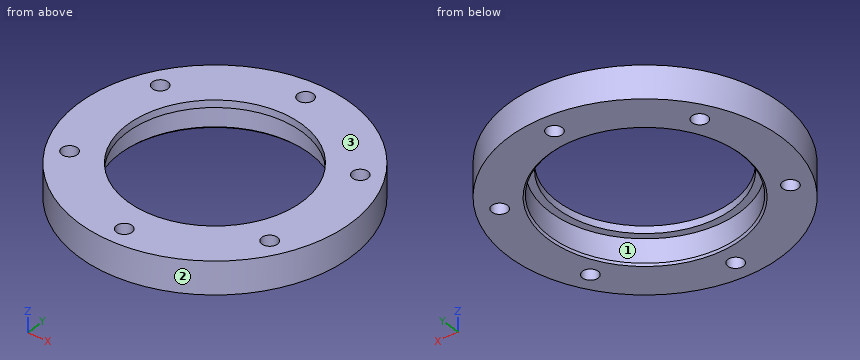
Autodesk Inventor part; units mm, degrees
ref_plane "YZ Plane" through (0, 0, 0) normal (1, 0, 0) x (0, 1, 0)
ref_plane "XZ Plane" through (0, 0, 0) normal (0, 1, 0) x (-1, 0, 0)
ref_plane "XY Plane" through (0, 0, 0) normal (0, 0, 1) x (1, 0, 0)
sketch "スケッチ1" plane through (0, 0, 0) normal (1, 0, 0) x (0, 1, 0)
  line L0 (24.1, 0) -> (24.1, -2)
  line L1 (24.1, -2) -> (26.1, -2)
  line L2 (26.1, -2) -> (26.1, -9)
  line L3 (26.1, -9) -> (37.5, -9)
  line L4 (37.5, -9) -> (37.5, 0)
  line L5 (37.5, 0) -> (24.1, 0)
  line L6 (0, -10.8) -> (0, 1.8)
  point P0 (0, 0)
  dimension "d0" = 26.1
  dimension "d1" = 37.5
  dimension "d2" = 7
  dimension "d3" = 2
  dimension "d4" = 2
revolve "回転1" add sketch "スケッチ1" angle 360 about axis through (0, 0, -10) along (0, 0, 1)
sketch "スケッチ2" plane through (0, 0, -9) normal (0, 0, -1) x (-1, 0, 0)
  circle A0 centre (0, 0) radius 32
  point P0 (0, 32)
  point P1 (-27.7128, 16)
  point P2 (-27.7128, -16)
  point P3 (0, -32)
  point P4 (27.7128, -16)
  point P5 (27.7128, 16)
  dimension "d6" = 64
  dimension "d9" = 360
hole "穴1" at (0, 32, -9) at (27.7128, 16, -9) at (27.7128, -16, -9) at (0, -32, -9) at (-27.7128, -16, -9) at (-27.7128, 16, -9) direction (0, 0, 1) diameter 4.3 end through all
chamfer "面取り1" distance 0.5 angle 45 1 edges at (0, -26.1, -9)
sketch "スケッチ3" plane through (0, 0, -9) normal (0, 0, -1) x (-1, 0, 0)
  circle A0 centre (-37.5, 0) radius 4.8
  circle A1 centre (0, 0) radius 37.5
  point P0 (-37.1928, 4.7902)
  point P1 (-37.1928, -4.7902)
  dimension "d18" = 9.6
properties part number "unit-base1" material "ABS プラスチック"
Geometry: final body of the model. Coordinates: model frame, mm. Face numbers are marked on the shaded views. Round coordinates to 2 decimals unless told otherwise and drop trailing zeros. Order: outer loops, then holes, each group sorted by start corner. A loop starts at its lowest first (then second) coordinate and runs counter-clockwise, first axis right, second up. Notation, with made-up numbers: M -22.75,17 L 23.25,17 A14 cw 23.25,33 Z; hole C -39.5,25 d8. An arc over 180 degrees is marked long. Use one line per item in the form item = value. Start each with the question number.
Q1. Cut plane D-D (y = -16). Count the separate pieces of the cut face and the enclosed holes in it, and give its area (3 significant figures).
Q2. Cut plane B-B (z = -6.5). Return loops of the section in (x, y).
Q3. Mould query, pull axis X, two halves, no side actions, for the marked faces 1, 2 and 3. Classes: +X half, -X half, draft (parallel to the pull), parting line (faces both ways), or undercut.
Q4. Cut plane C-C (y = -32). Return loops of the section in (x, z).
Q5. Material intervals for line 1 (Y direction, x = 0, z = -5); line 2 (X direction, y = -16, z = -2.25); line 3 (X direction, y = 0, z = -4.5), sorted ascending. Write a range as [from, to].
Q6. Cut plane A-A (y = 0). Return loops of the section in (x, z), and give its area (3 significant figures).
Q7. Pin query (flat end, axial travel): pin 1 Ø4 at (x, y) = (-27.71, 16) entering from +Z; pin 2 Ø4 at (x, z) = (-6.5, -1.5) entering from -Y; pin 3 Ø7 at (x, y) = (-27.71, -16) entering from -Z; pin 4 Ø1 at (x, z) = (9.5, -7) entering from -Y. Return the tip coordinate at first contact, or that it passes through.
Geometry results:
q1.separate_pieces = 4
q1.enclosed_holes = 0
q1.area = 172 mm^2
q2.outline = C 0,0 d75; hole C -27.71,-16 d4.3; hole C -27.71,16 d4.3; hole C 0,0 d52.2; hole C 0,-32 d4.3; hole C 0,32 d4.3; hole C 27.71,-16 d4.3; hole C 27.71,16 d4.3
q3.face_1 = undercut
q3.face_2 = parting line
q3.face_3 = draft
q4.outline = M -19.55,-9 L -2.15,-9 L -2.15,0 L -19.55,0 Z; M 2.15,-9 L 19.55,-9 L 19.55,0 L 2.15,0 Z
q5.line_1 = [-37.5, -34.15], [-29.85, -26.1], [26.1, 29.85], [34.15, 37.5]
q5.line_2 = [-33.92, -29.86], [-25.56, -20.62], [20.62, 25.56], [29.86, 33.92]
q5.line_3 = [-37.5, -26.1], [26.1, 37.5]
q6.outline = M -37.5,-9 L -26.6,-9 L -26.1,-8.5 L -26.1,-2 L -24.1,-2 L -24.1,0 L -37.5,0 Z; M 24.1,-2 L 26.1,-2 L 26.1,-8.5 L 26.6,-9 L 37.5,-9 L 37.5,0 L 24.1,0 Z
q6.area = 213 mm^2
q7.pin_1 = through
q7.pin_2 = -37.23
q7.pin_3 = -9
q7.pin_4 = -36.4
